Autodesk Inventor part; units mm, degrees
ref_plane "YZ Plane" through (0, 0, 0) normal (1, 0, 0) x (0, 1, 0)
ref_plane "XZ Plane" through (0, 0, 0) normal (0, 1, 0) x (-1, 0, 0)
ref_plane "XY Plane" through (0, 0, 0) normal (0, 0, 1) x (1, 0, 0)
sketch "Sketch1" plane through (0, 0, 0) normal (0, 1, 0) x (-1, 0, 0)
  line L0 (-75, 0) -> (-75, -100)
  line L1 (-75, -100) -> (75, -100)
  line L2 (75, -100) -> (75, 100)
  line L3 (75, 100) -> (-75, 100)
  line L4 (-75, 100) -> (-75, 0)
  circle A0 centre (69.4334, -94.4056) radius 3
  circle A1 centre (-69.396, -94.4056) radius 3
  circle A2 centre (-69.396, 94.4107) radius 3
  circle A3 centre (69.4334, 94.4107) radius 3
  point P0 (0, 0)
  dimension "d3" = 150
  dimension "d4" = 200
  dimension "d5" = 6
  dimension "d8" = 6
  dimension "d10" = 6
  dimension "d12" = 6
extrude "Extrusion1" add sketch "Sketch1" along normal blind 5
sketch "Sketch2" plane through (0, 5, 0) normal (0, 1, 0) x (1, 0, 0)
  circle A0 centre (-34.9985, -59.8752) radius 10
  circle A1 centre (35, -59.8759) radius 10
  line L0 (-35.1169, -34.8759) -> (-27.6169, -34.8759)
  line L1 (-27.6169, -34.8759) -> (-27.6169, -19.8759)
  line L2 (-27.6169, -19.8759) -> (-42.6169, -19.8759)
  line L3 (-42.6169, -19.8759) -> (-42.6169, -34.8759)
  line L4 (-42.6169, -34.8759) -> (-35.1169, -34.8759)
  line L5 (-27.6169, -37.8759) -> (-45.6169, -37.8759)
  line L6 (-45.6169, -37.8759) -> (-45.6169, -16.8759)
  line L7 (-45.6169, -16.8759) -> (-24.6169, -16.8759)
  line L8 (-24.6169, -16.8759) -> (-24.6169, -37.8759)
  line L9 (-24.6169, -37.8759) -> (-27.6169, -37.8759)
  line L10 (35, -34.8759) -> (42.5, -34.8759)
  line L11 (42.5, -34.8759) -> (42.5, -19.8759)
  line L12 (42.5, -19.8759) -> (27.5, -19.8759)
  line L13 (27.5, -19.8759) -> (27.5, -34.8759)
  line L14 (27.5, -34.8759) -> (35, -34.8759)
  line L15 (42.5, -37.8759) -> (24.5, -37.8759)
  line L16 (24.5, -37.8759) -> (24.5, -16.8759)
  line L17 (24.5, -16.8759) -> (45.5, -16.8759)
  line L18 (45.5, -16.8759) -> (45.5, -37.8759)
  line L19 (45.5, -37.8759) -> (42.5, -37.8759)
  line L20 (0, 85) -> (12.4518, 85)
  line L21 (12.4518, 85) -> (12.4518, 70)
  line L22 (12.4518, 70) -> (-12.5482, 70)
  line L23 (-12.5482, 70) -> (-12.5482, 85)
  line L24 (-12.5482, 85) -> (-0.0482, 85)
  line L25 (-12.5482, 85) -> (-12.5482, 77.5)
  circle A2 centre (-0.0482, 20) radius 6.5
  circle A3 centre (38, 20) radius 6.5
  line L26 (-75, 20) -> (-45, 20)
  circle A4 centre (-38.8669, 20) radius 6.5
  line L27 (12.4518, 67) -> (-15.5449, 67)
  line L28 (-15.5449, 67) -> (-15.5449, 88)
  line L29 (-15.5449, 88) -> (15.4551, 88)
  line L30 (15.4551, 88) -> (15.4551, 67)
  line L31 (15.4551, 67) -> (12.4518, 67)
  circle A5 centre (-18.5444, 77.4989) radius 3
  line L32 (-15.5449, 81.25) -> (-25.5449, 81.25)
  line L33 (-25.5449, 81.25) -> (-25.5449, 73.6405)
  line L34 (-25.5449, 73.6405) -> (-15.5449, 73.6405)
  circle A6 centre (18.4402, 77.4452) radius 3
  line L35 (15.4551, 73.6402) -> (25.4551, 73.6402)
  line L36 (25.4551, 73.6402) -> (25.4551, 81.25)
  line L37 (25.4551, 81.25) -> (15.4551, 81.25)
  line L38 (-12.5482, 85) -> (-15.5449, 85)
  line L39 (12.4518, 85) -> (15.4551, 85)
  line L40 (-12.5482, 85) -> (-12.5482, 88)
  line L41 (-12.5482, 70) -> (-12.5482, 67)
  line L42 (12.4518, 85) -> (12.4518, 88)
  line L43 (12.4518, 70) -> (12.4518, 67)
  line L44 (12.4518, 70) -> (15.4551, 70)
  line L45 (-12.5482, 70) -> (-15.5449, 70)
  point P0 (0, 0)
  point P1 (15.4551, 77.1464)
  point P2 (15.4551, 77.7441)
  point P3 (-15.5449, 77.5524)
  point P4 (-15.5449, 77.4455)
  dimension "d18" = 20
  dimension "d22" = 20
  dimension "d31" = 15
  dimension "d32" = 15
  dimension "d35" = 21
  dimension "d36" = 21
  dimension "d39" = 15
  dimension "d40" = 15
  dimension "d42" = 21
  dimension "d45" = 15
  dimension "d46" = 25
  dimension "d53" = 13
  dimension "d54" = 13
  dimension "d56" = 30
  dimension "d57" = 13
  dimension "d60" = 21
  dimension "d61" = 31
  dimension "d62" = 6
  dimension "d64" = 10
  dimension "d67" = 6
  dimension "d69" = 10
extrude "Extrusion2" add sketch "Sketch2" along normal blind 40 contours L42 L29 L30 L39
extrude "Extrusion3" add sketch "Sketch2" along normal blind 40 contours L39 L30 A6 L44 L21
extrude "Extrusion4" add sketch "Sketch2" along normal blind 40 contours L40 L38 L28 L29
extrude "Extrusion5" add sketch "Sketch2" along normal blind 40 contours L45 L28 L38 L23
extrude "Extrusion6" add sketch "Sketch2" along normal blind 40 contours L41 L27 L28 L45
extrude "Extrusion7" add sketch "Sketch2" along normal blind 40 contours L43 L27 L41 L22
extrude "Extrusion8" add sketch "Sketch2" along normal blind 40 contours L44 L30 L31 L43
extrude "Extrusion9" add sketch "Sketch2" along normal blind 40 contours L37 L36 L35 L30 A6
extrude "Extrusion10" add sketch "Sketch2" along normal blind 40 contours L34 L33 L32 L28
extrude "Extrusion11" add sketch "Sketch2" along normal blind 30 contours L5 L6 L7 L8 L9
extrude "Extrusion12" add sketch "Sketch2" along normal blind 30 contours L15 L16 L17 L18 L19
sketch "Sketch3" plane through (0, 5, 0) normal (0, 1, 0) x (1, 0, 0)
  circle A0 centre (-35, -59.8417) radius 10
  circle A1 centre (35, -60) radius 10
  circle A2 centre (0, 20) radius 5
  circle A3 centre (38, 20) radius 5
  circle A4 centre (-37, 20) radius 5
  circle A5 centre (0, 0) radius 5
  circle A6 centre (38, 0) radius 5
  circle A7 centre (-37, 0) radius 5
  dimension "d94" = 20
  dimension "d95" = 20
  dimension "d101" = 10
  dimension "d103" = 10
  dimension "d104" = 10
  dimension "d106" = 10
  dimension "d107" = 10
  dimension "d108" = 10
hole "Hole1" at (-35, 5, 59.8417) direction (0, -1, 0) diameter 20 end through all
hole "Hole2" at (35, 5, 60) direction (0, -1, 0) diameter 20 end through all
hole "Hole3" at (-37, 5, 0) direction (0, -1, 0) diameter 10 end through all
hole "Hole4" at (-37, 5, -20) direction (0, -1, 0) diameter 10 end through all
hole "Hole5" at (0, 5, -20) direction (0, -1, 0) diameter 10 end through all
hole "Hole6" at (0, 5, 0) direction (0, -1, 0) diameter 10 end through all
hole "Hole7" at (38, 5, -20) direction (0, -1, 0) diameter 10 end through all
hole "Hole8" at (38, 5, 0) direction (0, -1, 0) diameter 10 end through all
sketch "Sketch4" plane through (0, 5, 0) normal (0, 1, 0) x (1, 0, 0)
  circle A0 centre (0, 49) radius 7.5
  point P0 (0, 0)
  dimension "d166" = 15
hole "Hole9" at (0, 5, -49) direction (0, -1, 0) diameter 15 end through all
properties part number "Lock"
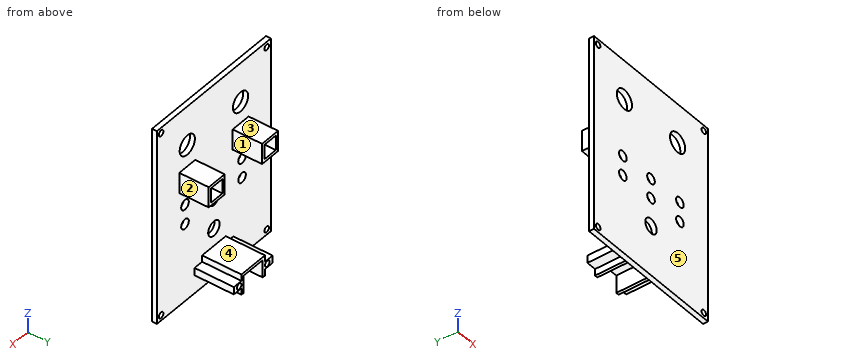
Can you work these out from the model? Positions are in its coordinate system, mm. Face numbers are marked on the shaded views. A direction names the side the tool comes from. Round coordinates to 2 decimals unless told otherwise and drop trailing zeros. Loops run counter-clockwise (first coordinate to the right, second up) from the corner with the lowest first, then second, coordinate; pieces in that order, holes last. Notation, with made-up numbers: (7.25, 82) - (42.25, 82) arc R29 ccw to (42.25, 107) - close; hole circle Ø2 at (53, 52). An arc over 180 degrees is marked (long way). Answer in a Markdown table with one row per item. Add a question column.
Q1. I want a section at C-C on x = 0. List the corners of the cut face in (y, z) for me.
Q2. I need wall thicknesses on L1, parallel to X at y = 9.5, z = 33.5; L2, parallel to Z at x = 28.5, y = 23; L3, parallel to X at y = 10, z = -86.5. Which ranges of each line are inside material? Lowest first, please.
Q3. I want a section at B-B on y = 29.5. Count the separate pieces of the cut face and the enclosed holes in it, and give its area (3 significant figures).
Q4. I want a section at D-D on z = -21.5. List the corners of the cut face in (x, y) for me, and give its area (3 significant figures).
Q5. For pin 1 Ø4.5 at (x, z) = (32, 28.5) entering from +Y; pin 2 Ø3.5 at (x, y) = (-14.5, 19.5) entering from -Z; pin 3 Ø2 at (y, z) = (15, -85) entering from +X, each with a flat end and sliding along its axis, tell me the tip position at first contact or that it passes through.
Q6. Which directions (+Z, -Z, +X, -X, +Y, -Y) give clear straight access to the entire face, cutting with the end or side of a thin tool? Please do the marked faces 4 and 5.
Q7. We'd pull the mould along X, two halves only. Please class the marked faces 1, 2 and 3: pulls with the +X half, pulls with the -X half, needs draft (parallel to the pull), parting line crosses it, or undercut.
Q8. I want a section at A-A on z = -49. List the corners of the cut face in (x, y) for me, and give its area (3 significant figures).
A:
| question | item | result |
|---|---|---|
| 1 | outline | (0, -100) - (5, -100) - (5, -70) - (45, -70) - (45, -67) - (5, -67) - (5, -56.5) - (0, -56.5) - close; (0, -41.5) - (5, -41.5) - (5, -25) - (0, -25) - close; (0, -15) - (5, -15) - (5, -5) - (0, -5) - close; (0, 5) - (5, 5) - (5, 100) - (0, 100) - close |
| 2 | L1 | -45.62 to -42.62, -27.62 to -24.62, 24.5 to 27.5, 42.5 to 45.5 |
| 2 | L2 | 16.88 to 19.88, 34.88 to 37.88 |
| 2 | L3 | -15.54 to -12.55, 12.45 to 15.46 |
| 3 | separate pieces | 3 |
| 3 | enclosed holes | 4 |
| 3 | area | 729 mm^2 |
| 4 | outline | (-75, 0) - (-41.77, 0) - (-41.77, 5) - (-75, 5) - close; (-32.23, 0) - (-4.77, 0) - (-4.77, 5) - (-32.23, 5) - close; (4.77, 0) - (33.23, 0) - (33.23, 5) - (4.77, 5) - close; (42.77, 0) - (75, 0) - (75, 5) - (42.77, 5) - close |
| 4 | area | 607 mm^2 |
| 5 | pin 1 | y = 5 |
| 5 | pin 2 | z = -88 |
| 5 | pin 3 | x = 15.46 |
| 6 | face 4 | +Z, +X, -X, +Y |
| 6 | face 5 | +Z, -Z, +X, -X, -Y |
| 7 | face 1 | undercut |
| 7 | face 2 | pulls with the +X half |
| 7 | face 3 | needs draft |
| 8 | outline | (-75, 0) - (-7.5, 0) - (-7.5, 5) - (-75, 5) - close; (7.5, 0) - (75, 0) - (75, 5) - (7.5, 5) - close |
| 8 | area | 675 mm^2 |
